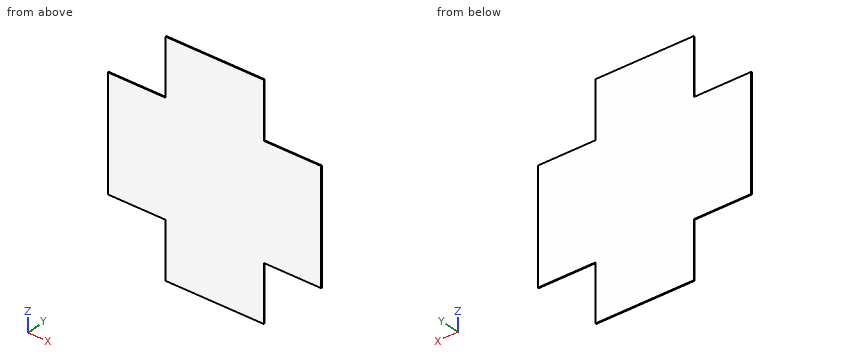
```python
from build123d import *

# Parameters (mm, degrees)
SKETCH1_W           = 177.8
SKETCH1_H           = 355.6
SKETCH1_W_2         = 304.8
SKETCH1_H_2         = 177.8
BOSS_EXTRUDE1_DEPTH = 1.5875


with BuildPart() as part:
    # Sketch1 → Boss-Extrude1 (new, symmetric)
    with BuildSketch(Plane(origin=(0, 0, 0), x_dir=(1, 0, 0), z_dir=(0, 1, 0))):
        with Locations((-241.3, 0)):
            Rectangle(SKETCH1_W, SKETCH1_H)
        Rectangle(SKETCH1_W_2, SKETCH1_H)
        with Locations((0, 266.7)):
            Rectangle(SKETCH1_W_2, SKETCH1_H_2)
        with Locations((0, -266.7)):
            Rectangle(SKETCH1_W_2, SKETCH1_H_2)
        with Locations((241.3, 0)):
            Rectangle(SKETCH1_W, SKETCH1_H)
    extrude(amount=BOSS_EXTRUDE1_DEPTH, both=True)


solid = part.part
```
The listing builds one solid part. Answer for the finished solid, in the listing's coordinates (mm). Give positions to 0.01 mm unless a question says otherwise; leave off trailing zeros. Order: outer loops, then holes, each group sorted by start corner. A loop starts at its lowest first (then second) coordinate and runs counter-clockwise, first axis right, second up. Notation, with made-up numbers: (50, 39) - (100, 39) arc R19 ccw to (100, 44) - close; hole circle Ø7 at (14.5, 57.5). An arc over 180 degrees is marked (long way). Answer in a Markdown table with one row per item. Add a question column.
Q1. The part is cut by section B-B (x = 242.5). Determine the outline of the cut face in (y, z).
Q2. Find the intervals of material crossed by line 1 along Z through (x, y) = (-246.5, -1.15); line 2 along X through (y, z) = (-0.75, -273), in increasing order. Write a range as [from, to].
Q3. The part is cut by section A-A (y = 0.75). Determine the outline of the cut face in (x, z), then the cut area to 3 significant figures.
Q4. Given P1, Ø1, axis at x = -211, y = 0, coming from the +Z side; P2, Ø1.6, axis at x = 202, y = -0.5, coming from the -Z side; P3, Ø1.6, axis at y = -0.5, z = 243.5, coming from the +X side, each flat-ended and moving along its own axis, determine where each tip first touches the part or whether it passes through.
Q5. The part is cut by section C-C (z = 298.5). Determine the outline of the cut face in (x, y).
Determined:
| question | item | result |
|---|---|---|
| 1 | outline | (-1.59, -177.8) - (1.59, -177.8) - (1.59, 177.8) - (-1.59, 177.8) - close |
| 2 | line 1 | z = [-177.8, 177.8] |
| 2 | line 2 | x = [-152.4, 152.4] |
| 3 | outline | (-330.2, -177.8) - (-152.4, -177.8) - (-152.4, -355.6) - (152.4, -355.6) - (152.4, -177.8) - (330.2, -177.8) - (330.2, 177.8) - (152.4, 177.8) - (152.4, 355.6) - (-152.4, 355.6) - (-152.4, 177.8) - (-330.2, 177.8) - close |
| 3 | area | 343,000 mm² |
| 4 | P1 | stops at z = 177.8 |
| 4 | P2 | stops at z = -177.8 |
| 4 | P3 | stops at x = 152.4 |
| 5 | outline | (-152.4, -1.59) - (152.4, -1.59) - (152.4, 1.59) - (-152.4, 1.59) - close |
